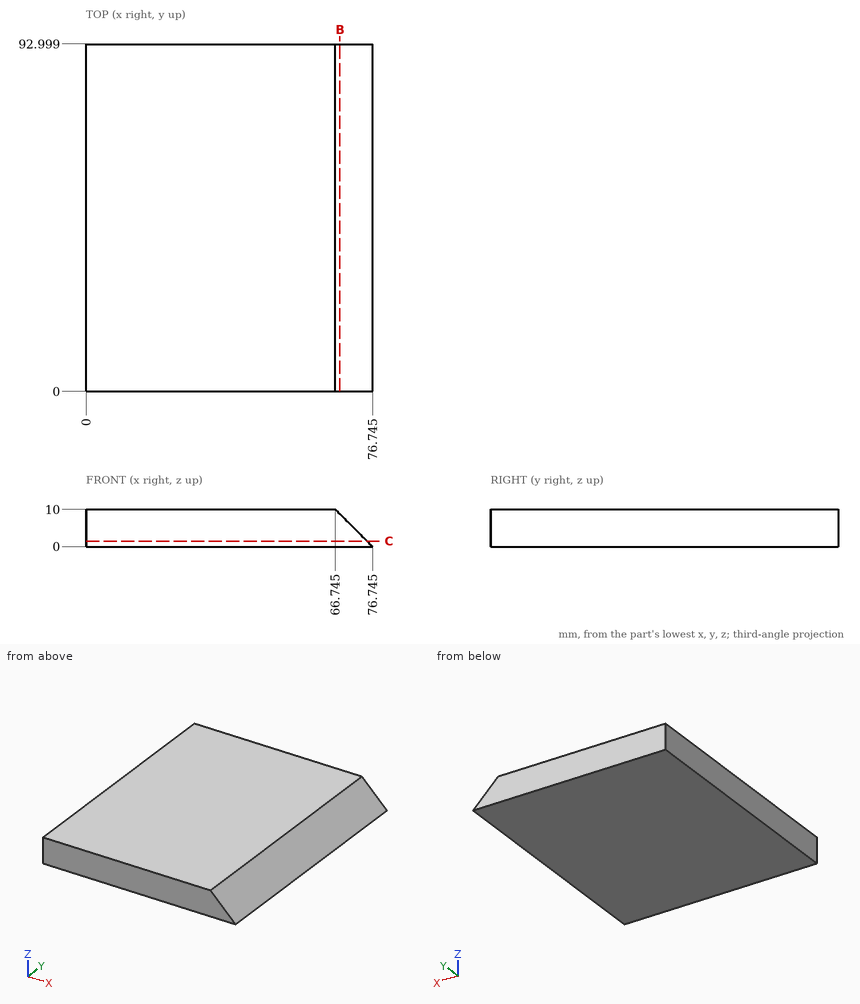
Drawing for the job (mm, zero at the part's lowest x, y, z). Coordinates: 2 decimals unless noted, no trailing zeros. Order: outer loops, then holes, each group sorted by start corner. A loop starts at its lowest first (then second) coordinate and runs counter-clockwise, first axis right, second up. Notation, with made-up numbers: (33, -29.5) -> (58, -29.5) arc R29 ccw to (58, -1.5) -> close; hole circle Ø10 at (-14.5, 77.25). An arc over 180 degrees is marked (long way). One line per item, written item: value.
(1) Slice it at C-C, the plane z = 1.5. List the corners of the cut face in (x, y) (1 decimal), plus the area to 3 significant figures.
Checked values:
outline: (0, 0) -> (75.2, 0) -> (75.2, 93) -> (0, 93) -> close
area: 7,000 mm2
(2) Slice it at B-B, the plane x = 68. List the corners of the cut face in (y, z) (1 decimal), plus the area to 3 significant figures.
Checked values:
outline: (0, 0) -> (93, 0) -> (93, 8.7) -> (0, 8.7) -> close
area: 813 mm2
(3) Probe line 1 (Z direction, x = 72, y = 72.5) (1 decimal); line 2 (X direction, y = 30.5, z = 8) (1 decimal); line 3 (X direction, y = 51, z = 5.25) (1 decimal). List the from-to ranges inside material, lowest first. Write a range as [from, to].
Checked values:
line 1: [0, 4.7]
line 2: [0, 68.7]
line 3: [0, 71.5]
(4) Drop flat-ended pins along their axis: pin 1 Ø1.5 at (x, z) = (12, 1.5) entering from -Y; pin 2 Ø1 at (y, z) = (69.5, 7.5) entering from +X (1 decimal). Give the stop position or say it passes through.
Checked values:
pin 1: y = 0
pin 2: x = 69.7
